Part model, mm, in its own coordinate system. A direction names the side the tool comes from. Coordinates: 2 decimals unless noted, no trailing zeros. Order: outer loops, then holes, each group sorted by start corner. A loop starts at its lowest first (then second) coordinate and runs counter-clockwise, first axis right, second up.
Autodesk Inventor part; units mm, degrees
ref_plane "YZ Plane" through (0, 0, 0) normal (1, 0, 0) x (0, 1, 0)
ref_plane "XZ Plane" through (0, 0, 0) normal (0, 1, 0) x (-1, 0, 0)
ref_plane "XY Plane" through (0, 0, 0) normal (0, 0, 1) x (1, 0, 0)
sketch "Sketch_1" plane through (0, 0, 0) normal (0, 0, 1) x (1, 0, 0)
  line L0 (12, 0) -> (-3, 0)
  line L1 (-3, 0) -> (-3, 2.45)
  line L2 (-3, 2.45) -> (-2.7, 2.75)
  line L3 (-2.7, 2.75) -> (0, 2.75)
  line L4 (0, 2.75) -> (0, 1.5)
  line L5 (0, 1.5) -> (11.6935, 1.5)
  line L6 (11.6935, 1.5) -> (12, 1.1935)
  line L7 (12, 1.1935) -> (12, 0)
  line L8 (12, 0) -> (-3, 0)
revolve "Revolution1" add sketch "Sketch_1" angle 360 about axis through (12, 0, 0) along (1, 0, 0)
thread "Thread1"
sketch "Sketch_2" plane through (-3, 0, 0) normal (1, 0, 0) x (0, 0, -1)
  line L0 (-1.25, -0.7217) -> (0, -1.4434)
  line L1 (0, -1.4434) -> (1.25, -0.7217)
  line L2 (1.25, -0.7217) -> (1.25, 0.7217)
  line L3 (1.25, 0.7217) -> (0, 1.4434)
  line L4 (0, 1.4434) -> (-1.25, 0.7217)
  line L5 (-1.25, 0.7217) -> (-1.25, -0.7217)
extrude "Extrusion1" cut sketch "Sketch_2" along normal blind 1.8
properties part number "SNSX-M3-12-88"
Q1. Pin check, flat tips, straight feed: pin 1 Ø1.2 at (x, y) = (-2, 0.5) entering from +Z; pin 2 Ø1.5 at (x, z) = (3, -1.5) entering from -Y; pin 3 Ø1 at (x, z) = (1, -1.5) entering from -Y; pin 4 Ø2 at (x, y) = (4.5, 0) entering from +Z. Stop position of each tip, or through.
Results list:
pin 1: stops at z = 2.75
pin 2: stops at y = -1.3
pin 3: stops at y = -1.12
pin 4: stops at z = 1.5
Q2. Mould opens along Y. For faces 4 (the face through (-2.11, -1.08, 0.63)), 5 (the face through (-1.331, -0.596, -2.685)), 6 (the face through (0, 1.2, -1.2)) say: pulls with the +Y half, pulls with the -Y half, needs draft (parallel to the pull), parting line crosses it, or undercut.
Results list:
face 4: undercut
face 5: parting line crosses it
face 6: needs draft
Q3. Cut at A-A on y = 0. Write the cut outline in (x, z), and give its area (3 significant figures).
Results list:
outline: (-3, -2.45) - (-2.7, -2.75) - (0, -2.75) - (0, -1.5) - (11.69, -1.5) - (12, -1.19) - (12, 1.19) - (11.69, 1.5) - (0, 1.5) - (0, 2.75) - (-2.7, 2.75) - (-3, 2.45) - (-3, 1.25) - (-1.2, 1.25) - (-1.2, -1.25) - (-3, -1.25) - close
area: 47.8 mm2
Q4. Wall check: line 1 along X through (y, z) = (1.5, 1.7); line 2 along X through (y, z) = (-1, 0); line 3 along Y through (x, z) = (11, -0.65). Give the ranges that are in metal, low to high.
Results list:
line 1: x = -3 to 0
line 2: x = -1.2 to 12
line 3: y = -1.35 to 1.35
Q5. Cut at B-B on x = 2.5. Write the cut outline in (y, z).
Results list:
outline: circle Ø3 at (0, 0)
Q6. Which spindle directions (+Z, -Z, +X, -X, +Y, -Y) get a long thin tool onto all of the face, cutting with end or side? Do faces 1 (the face through (5.93, -1.5, 0.07)), 2 (the face through (12, 0, 0)), 3 (the face through (-2.11, 1.08, -0.63)). Say none if no direction does.
Results list:
face 1: +X
face 2: +Z, -Z, +X, +Y, -Y
face 3: -X
